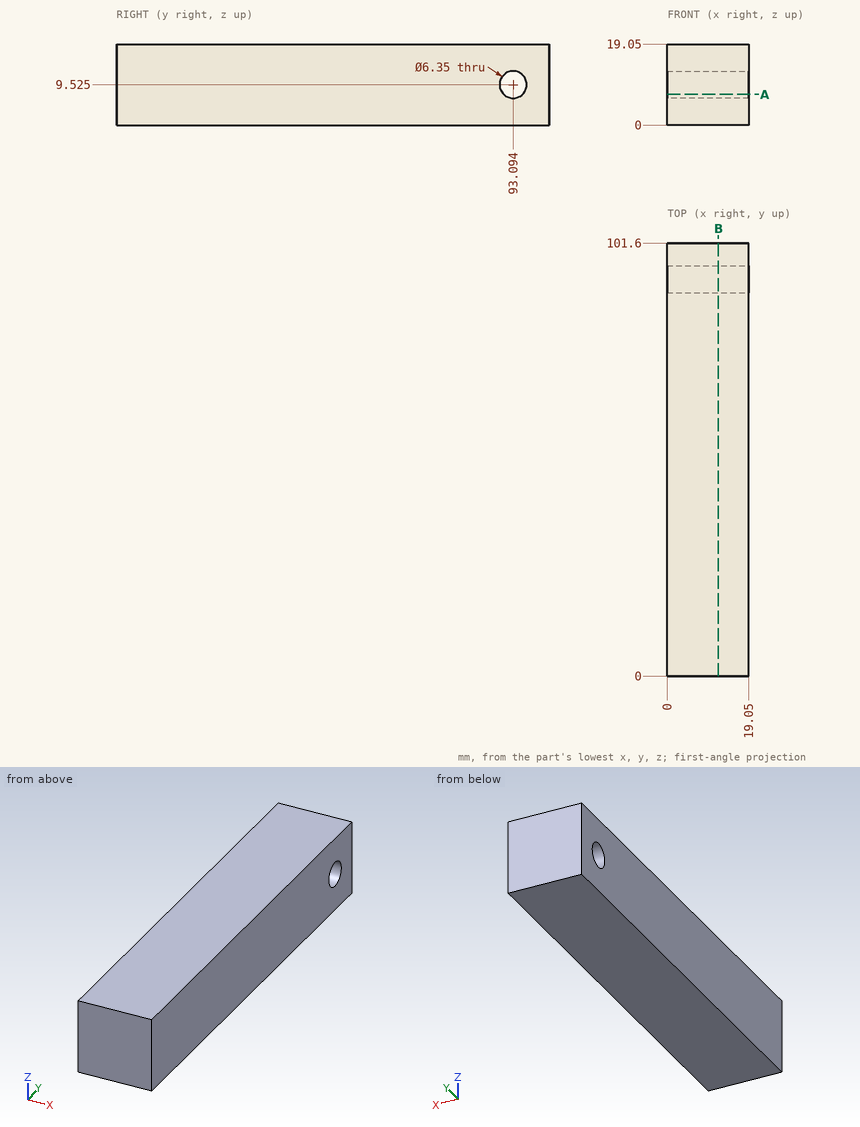
Input: dimensioned drawing with shaded views. Units: mm. Origin: part minimum x, y, z. Coordinates: 2 decimals unless noted, no trailing zeros. Write each loop counter-clockwise with the first axis right and the second up, starting at its lowest first coordinate (ties: lowest second). Pieces come first, ordered by that corner, then holes. Notation, with made-up numbers: M 83,18.5 L 141,18.5 A22 cw 141,31.5 Z; hole C -31,50 d11. An arc over 180 degrees is marked long. Use a Markdown table: item, result.
1) Section A-A, the plane z = 7.25. Output: boundary loops of the cut face in (x, y), then the cut area to 3 significant figures.
Conclusion:
| item | result |
|---|---|
| outline | M 0,0 L 19.05,0 L 19.05,90.88 L 0,90.88 Z; M 0,95.31 L 19.05,95.31 L 19.05,101.6 L 0,101.6 Z |
| area | 1,850 mm^2 |
2) Section B-B, the plane x = 12. Output: boundary loops of the cut face in (y, z) (3 decimals), then the cut area to 3 significant figures.
Conclusion:
| item | result |
|---|---|
| outline | M 0,0 L 101.6,0 L 101.6,19.05 L 0,19.05 Z; hole C 93.094,9.525 d6.35 |
| area | 1,900 mm^2 |
3) Ray query, L1, parallel to Z at x = 4, y = 95; L2, parallel to Y at x = 4.5, z = 11.5; L3, parallel to Y at x = 15.5, z = 8.5. Return the intervals inside material, ascending.
Conclusion:
| item | result |
|---|---|
| L1 | z = 0 to 6.99, 12.06 to 19.05 |
| L2 | y = 0 to 90.61, 95.58 to 101.6 |
| L3 | y = 0 to 90.09, 96.1 to 101.6 |
